```python
from build123d import *

# Parameters (mm, degrees)
BOSS_EXTRUDE1_DEPTH = 400


with BuildPart() as part:
    # Sketch1 → Boss-Extrude1 (new body)
    with BuildSketch(Plane(origin=(0, 0, 0), x_dir=(1, 0, 0), z_dir=(0, 1, 0))):
        with BuildLine():
            ThreePointArc((-4.185606061, -4.972997276), (0, -6.5), (4.185606061, -4.972997276))
            ThreePointArc((4.185606061, -4.972997276), (4.532194193, -4.345235079), (4.369444444, -3.646864669))
            ThreePointArc((4.369444444, -3.646864669), (3.25, 0), (4.369444444, 3.646864669))
            ThreePointArc((4.369444444, 3.646864669), (4.532194193, 4.345235079), (4.185606061, 4.972997276))
            ThreePointArc((4.185606061, 4.972997276), (0, 6.5), (-4.185606061, 4.972997276))
            ThreePointArc((-4.185606061, 4.972997276), (-4.532194193, 4.345235079), (-4.369444444, 3.646864669))
            ThreePointArc((-4.369444444, 3.646864669), (-3.25, 0), (-4.369444444, -3.646864669))
            ThreePointArc((-4.369444444, -3.646864669), (-4.532194193, -4.345235079), (-4.185606061, -4.972997276))
        make_face()
        with BuildLine():
            ThreePointArc((-3.055555556, -4.573136806), (0, -5.5), (3.055555556, -4.573136806))
            ThreePointArc((3.055555556, -4.573136806), (3.473728991, -3.969367404), (3.366666667, -3.242769735))
            ThreePointArc((3.366666667, -3.242769735), (2.5, 0), (3.366666667, 3.242769735))
            ThreePointArc((3.366666667, 3.242769735), (3.473728991, 3.969367404), (3.055555556, 4.573136806))
            ThreePointArc((3.055555556, 4.573136806), (0, 5.5), (-3.055555556, 4.573136806))
            ThreePointArc((-3.055555556, 4.573136806), (-3.473728991, 3.969367404), (-3.366666667, 3.242769735))
            ThreePointArc((-3.366666667, 3.242769735), (-2.5, 0), (-3.366666667, -3.242769735))
            ThreePointArc((-3.366666667, -3.242769735), (-3.473728991, -3.969367404), (-3.055555556, -4.573136806))
        make_face(mode=Mode.SUBTRACT)
    extrude(amount=BOSS_EXTRUDE1_DEPTH)


solid = part.part
```
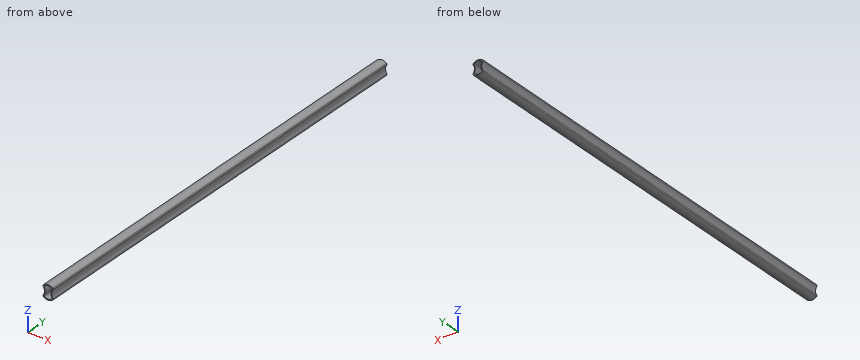
Work out the finished part from the listing and answer in its coordinate system (mm). Round coordinates to 2 decimals unless told otherwise and drop trailing zeros. Loops run counter-clockwise (first coordinate to the right, second up) from the corner with the lowest first, then second, coordinate; pieces in that order, holes last. Notation, with made-up numbers: (73.25, -5) -> (102.25, -5) arc R32 cw to (102.25, 33) -> close; hole circle Ø3 at (74, 36.5). An arc over 180 degrees is marked (long way). Write each question's results on one line, items separated by ' | '. Start each with the question number.
1. Find the intervals of material crossed by probe 1 along X at (y, z) = (356, 0.75); probe 2 along X at (y, z) = (308, -4.25); probe 3 along X at (y, z) = (298.5, -5.75), in increasing order. Write a range as from..to.
2. Section A-A (x = -1) is taken. Determine the outline of the cut face in (y, z), plus the area to 3 significant figures.
3. Section C-C (z = -0.75) is taken. Determine the outline of the cut face in (x, y), plus the area to 3 significant figures.
4. Given pin 1 Ø1 at (x, y) = (-3.5, 139) entering from -Z; pin 2 Ø5 at (y, z) = (163.5, -1.5) entering from -X, each flat-ended and moving along its own axis, determine where each tip first touches the part or whether it passes through.
5. Section B-B (y = 73) is taken. Determine the outline of the cut face in (x, z).
Evaluation:
1) probe 1: x = -3.29..-2.54, 2.54..3.29 | probe 2: x = -4.54..-3.36, 3.36..4.54 | probe 3: x = -3.03..3.03
2) outline: (0, -6.42) -> (400, -6.42) -> (400, -5.41) -> (0, -5.41) -> close; (0, 5.41) -> (400, 5.41) -> (400, 6.42) -> (0, 6.42) -> close | area: 811 mm2
3) outline: (-3.29, 0) -> (-2.54, 0) -> (-2.54, 400) -> (-3.29, 400) -> close; (2.54, 0) -> (3.29, 0) -> (3.29, 400) -> (2.54, 400) -> close | area: 600 mm2
4) pin 1: stops at z = -5.77 | pin 2: stops at x = -4.52
5) outline: (-4.37, -3.65) arc R1 ccw to (-4.19, -4.97) arc R6.5 ccw to (4.19, -4.97) arc R1 ccw to (4.37, -3.65) arc R6.5 cw to (4.37, 3.65) arc R1 ccw to (4.19, 4.97) arc R6.5 ccw to (-4.19, 4.97) arc R1 ccw to (-4.37, 3.65) arc R6.5 cw to start; hole (-3.37, -3.24) arc R1 ccw to (-3.06, -4.57) arc R5.5 ccw to (3.06, -4.57) arc R1 ccw to (3.37, -3.24) arc R6.5 cw to (3.37, 3.24) arc R1 ccw to (3.06, 4.57) arc R5.5 ccw to (-3.06, 4.57) arc R1 ccw to (-3.37, 3.24) arc R6.5 cw to start
